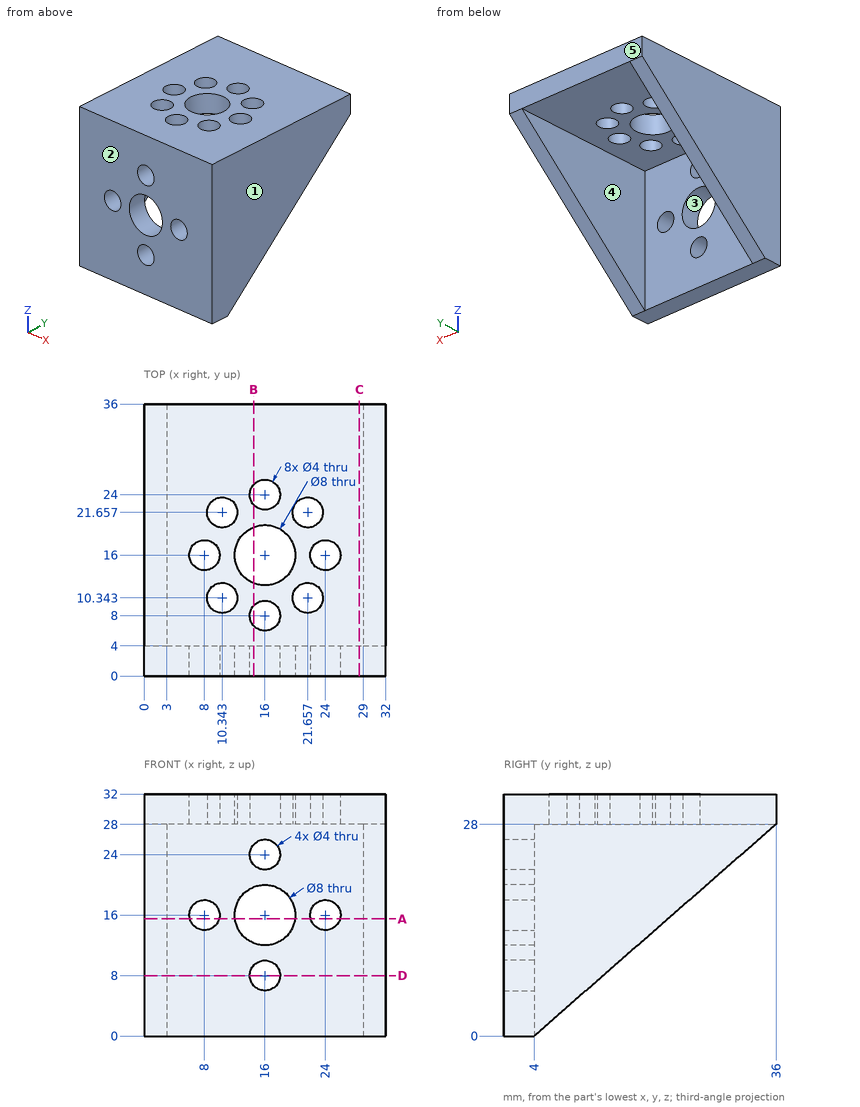
Could you check a few things on this drawing? It's one solid part, dimensions in mm from its lowest x, y, z. A direction names the side the tool comes from. Coordinates: 2 decimals unless noted, no trailing zeros. Write each loop counter-clockwise with the first axis right and the second up, starting at its lowest first coordinate (ties: lowest second). Pieces come first, ordered by that corner, then holes.
1) If I drill on line 1 (X direction, y = 2.5, z = 8); line 2 (X direction, y = 18, z = 24); line 3 (Z direction, x = 9.5, y = 33), over which ranges is the centre line in solid material (lowest first)?
Filled in:
line 1: x = 0 to 14, 18 to 32
line 2: x = 0 to 3, 29 to 32
line 3: z = 28 to 32
2) If we section it at C-C (x = 28.5): List the corners of the cut face in (y, z) for me, plus the area to 3 significant figures.
Filled in:
outline: (0, 0) - (4, 0) - (4, 28) - (36, 28) - (36, 32) - (0, 32) - close
area: 256 mm2
3) I'm going to push flat-ended pins straight in: pin 1 (6.5 mm diameter, centred on x = 24, y = 16, fed in from -Z); pin 2 (10.5 mm diameter, centred on x = 16, z = 16, fed in from +Y); pin 3 (3.5 mm diameter, centred on x = 8, z = 16, fed in from +Y). Where does each tip first touch, or does it pass through?
Filled in:
pin 1: stops at z = 28
pin 2: stops at y = 4
pin 3: passes through
4) Thinking about a two-plate mould opening in X: for the marked faces 1, 2 and 3, which applies, +X half, -X half, draft (parallel to the pull), parting line (faces both ways), or undercut?
Filled in:
face 1: +X half
face 2: draft
face 3: undercut
5) If we section it at D-D (z = 8): List the corners of the cut face in (x, y) for me.
Filled in:
outline: (0, 0) - (14, 0) - (14, 4) - (3, 4) - (3, 13.14) - (0, 13.14) - close; (18, 0) - (32, 0) - (32, 13.14) - (29, 13.14) - (29, 4) - (18, 4) - close
6) If we section it at B-B (x = 14.5): Count the separate pieces of the cut face and the enclosed holes in it, plus the area to 3 significant figures.
Filled in:
separate pieces: 7
enclosed holes: 0
area: 154 mm2
7) If we section it at A-A (z = 15.5): List the corners of the cut face in (x, y) for me, plus the area to 3 significant figures.
Filled in:
outline: (0, 0) - (6.06, 0) - (6.06, 4) - (3, 4) - (3, 21.71) - (0, 21.71) - close; (9.94, 0) - (12.03, 0) - (12.03, 4) - (9.94, 4) - close; (19.97, 0) - (22.06, 0) - (22.06, 4) - (19.97, 4) - close; (25.94, 0) - (32, 0) - (32, 21.71) - (29, 21.71) - (29, 4) - (25.94, 4) - close
area: 172 mm2
8) Which directions (+Z, -Z, +X, -X, +Y, -Y) give clear straight access to the entire face, cutting with the end or side of a thin tool? Please do the marked faces 4 and 5.
Filled in:
face 4: -Z, +Y
face 5: +Z, -Z, +X, -X, +Y
